For this review, take the finished solid that the model builds, in its own axes (mm). Coordinates: 2 decimals unless noted, no trailing zeros. Loops run counter-clockwise (first coordinate to the right, second up) from the corner with the lowest first, then second, coordinate; pieces in that order, holes last. Notation, with made-up numbers: (67, 24) - (99, 24) arc R24 cw to (99, 58) - close; hole circle Ø5 at (11, 49.25). An arc over 180 degrees is marked (long way). One line per item, written item: value. Start each with the question number.
1. Take a section at B-B, the plane x = 5. Count the separate pieces of the cut face and the enclosed holes in it, and give its area (3 significant figures).
2. Take a section at A-A, the plane y = 31.5. State the section outline as (x, z) points.
3. To check wall thickness, follow line 1 (Y direction, x = -29.5, z = 2.05). State the ranges of the line that lie inside material, in increasing order. Write a range as from..to.
4. Take a section at D-D, the plane x = -28.5. State the section outline as (y, z) points, and give its area (3 significant figures).
5. The part is to be moulded in two halves that separate along Y. For faces 1 (the face through (-5, 49, 1)), 2 (the face through (-15, -58, 1)), say which applies: released by +Y, released by -Y, zero draft, split by the parting line, or undercut.
6. Insertion check: pin 1 (1 mm diameter, centred on x = 25, z = 2.5, fed in from -Y); pin 2 (0.9 mm diameter, centred on y = 58.5, z = 1, fed in from +X). Each pin has a flat end and moves straight along its axis. Give the tip position at first contact, or say it passes through.
```python
from build123d import *

# Parameters (mm, degrees)
SKETCH1_R           = 1.5
BOSS_EXTRUDE1_DEPTH = 3


with BuildPart() as part:
    # Sketch1 → Boss-Extrude1 (new body)
    with BuildSketch(Plane.XY):
        Polygon((-35, 56.5), (-35, -56.5), (-15, -56.5), (-15, -59.5), (15, -59.5), (15, -56.5), (35, -56.5), (35, 56.5), (25, 56.5), (15, 56.5), (15, 59.5), (5, 59.5), (-5, 59.5), (-15, 59.5), (-15, 56.5), (-25, 56.5), align=None)
        with Locations((-25, 51.5)):
            Circle(SKETCH1_R, mode=Mode.SUBTRACT)
        with Locations((-25, 41.5)):
            Circle(SKETCH1_R, mode=Mode.SUBTRACT)
        with Locations((-25, 31.5)):
            Circle(SKETCH1_R, mode=Mode.SUBTRACT)
        with Locations((-25, 21.5)):
            Circle(SKETCH1_R, mode=Mode.SUBTRACT)
        with Locations((-25, 11.5)):
            Circle(SKETCH1_R, mode=Mode.SUBTRACT)
        with Locations((-25, 3.5)):
            Circle(SKETCH1_R, mode=Mode.SUBTRACT)
        with Locations((-25, -3.5)):
            Circle(SKETCH1_R, mode=Mode.SUBTRACT)
        with Locations((-25, -11.5)):
            Circle(SKETCH1_R, mode=Mode.SUBTRACT)
        with Locations((-25, -21.5)):
            Circle(SKETCH1_R, mode=Mode.SUBTRACT)
        with Locations((-25, -31.5)):
            Circle(SKETCH1_R, mode=Mode.SUBTRACT)
        with Locations((-25, -51.5)):
            Circle(SKETCH1_R, mode=Mode.SUBTRACT)
        with Locations((-15, 51.5)):
            Circle(SKETCH1_R, mode=Mode.SUBTRACT)
        with Locations((-15, 41.5)):
            Circle(SKETCH1_R, mode=Mode.SUBTRACT)
        with Locations((-15, 31.5)):
            Circle(SKETCH1_R, mode=Mode.SUBTRACT)
        with Locations((-15, 21.5)):
            Circle(SKETCH1_R, mode=Mode.SUBTRACT)
        with Locations((-15, 11.5)):
            Circle(SKETCH1_R, mode=Mode.SUBTRACT)
        with Locations((-15, 3.5)):
            Circle(SKETCH1_R, mode=Mode.SUBTRACT)
        with Locations((-15, -3.5)):
            Circle(SKETCH1_R, mode=Mode.SUBTRACT)
        with Locations((-15, -11.5)):
            Circle(SKETCH1_R, mode=Mode.SUBTRACT)
        with Locations((-15, -21.5)):
            Circle(SKETCH1_R, mode=Mode.SUBTRACT)
        with Locations((-15, -31.5)):
            Circle(SKETCH1_R, mode=Mode.SUBTRACT)
        with Locations((-15, -51.5)):
            Circle(SKETCH1_R, mode=Mode.SUBTRACT)
        with Locations((-5, 50.5)):
            Circle(SKETCH1_R, mode=Mode.SUBTRACT)
        with Locations((-5, 41.5)):
            Circle(SKETCH1_R, mode=Mode.SUBTRACT)
        with Locations((-5, 31.5)):
            Circle(SKETCH1_R, mode=Mode.SUBTRACT)
        with Locations((-5, 21.5)):
            Circle(SKETCH1_R, mode=Mode.SUBTRACT)
        with Locations((-5, 11.5)):
            Circle(SKETCH1_R, mode=Mode.SUBTRACT)
        with Locations((-5, 3.5)):
            Circle(SKETCH1_R, mode=Mode.SUBTRACT)
        with Locations((-5, -3.5)):
            Circle(SKETCH1_R, mode=Mode.SUBTRACT)
        with Locations((-5, -11.5)):
            Circle(SKETCH1_R, mode=Mode.SUBTRACT)
        with Locations((-5, -21.5)):
            Circle(SKETCH1_R, mode=Mode.SUBTRACT)
        with Locations((-5, -31.5)):
            Circle(SKETCH1_R, mode=Mode.SUBTRACT)
        with Locations((-5, -51.5)):
            Circle(SKETCH1_R, mode=Mode.SUBTRACT)
        with Locations((5, 50.5)):
            Circle(SKETCH1_R, mode=Mode.SUBTRACT)
        with Locations((5, 41.5)):
            Circle(SKETCH1_R, mode=Mode.SUBTRACT)
        with Locations((5, 31.5)):
            Circle(SKETCH1_R, mode=Mode.SUBTRACT)
        with Locations((5, 21.5)):
            Circle(SKETCH1_R, mode=Mode.SUBTRACT)
        with Locations((5, 11.5)):
            Circle(SKETCH1_R, mode=Mode.SUBTRACT)
        with Locations((5, 3.5)):
            Circle(SKETCH1_R, mode=Mode.SUBTRACT)
        with Locations((5, -3.5)):
            Circle(SKETCH1_R, mode=Mode.SUBTRACT)
        with Locations((5, -11.5)):
            Circle(SKETCH1_R, mode=Mode.SUBTRACT)
        with Locations((5, -21.5)):
            Circle(SKETCH1_R, mode=Mode.SUBTRACT)
        with Locations((5, -31.5)):
            Circle(SKETCH1_R, mode=Mode.SUBTRACT)
        with Locations((5, -51.5)):
            Circle(SKETCH1_R, mode=Mode.SUBTRACT)
        with Locations((15, 51.5)):
            Circle(SKETCH1_R, mode=Mode.SUBTRACT)
        with Locations((15, 41.5)):
            Circle(SKETCH1_R, mode=Mode.SUBTRACT)
        with Locations((15, 31.5)):
            Circle(SKETCH1_R, mode=Mode.SUBTRACT)
        with Locations((15, 21.5)):
            Circle(SKETCH1_R, mode=Mode.SUBTRACT)
        with Locations((15, 11.5)):
            Circle(SKETCH1_R, mode=Mode.SUBTRACT)
        with Locations((15, 3.5)):
            Circle(SKETCH1_R, mode=Mode.SUBTRACT)
        with Locations((15, -3.5)):
            Circle(SKETCH1_R, mode=Mode.SUBTRACT)
        with Locations((15, -11.5)):
            Circle(SKETCH1_R, mode=Mode.SUBTRACT)
        with Locations((15, -21.5)):
            Circle(SKETCH1_R, mode=Mode.SUBTRACT)
        with Locations((15, -31.5)):
            Circle(SKETCH1_R, mode=Mode.SUBTRACT)
        with Locations((15, -51.5)):
            Circle(SKETCH1_R, mode=Mode.SUBTRACT)
        with Locations((25, 51.5)):
            Circle(SKETCH1_R, mode=Mode.SUBTRACT)
        with Locations((25, 41.5)):
            Circle(SKETCH1_R, mode=Mode.SUBTRACT)
        with Locations((25, 31.5)):
            Circle(SKETCH1_R, mode=Mode.SUBTRACT)
        with Locations((25, 21.5)):
            Circle(SKETCH1_R, mode=Mode.SUBTRACT)
        with Locations((25, 11.5)):
            Circle(SKETCH1_R, mode=Mode.SUBTRACT)
        with Locations((25, 3.5)):
            Circle(SKETCH1_R, mode=Mode.SUBTRACT)
        with Locations((25, -3.5)):
            Circle(SKETCH1_R, mode=Mode.SUBTRACT)
        with Locations((25, -11.5)):
            Circle(SKETCH1_R, mode=Mode.SUBTRACT)
        with Locations((25, -21.5)):
            Circle(SKETCH1_R, mode=Mode.SUBTRACT)
        with Locations((25, -31.5)):
            Circle(SKETCH1_R, mode=Mode.SUBTRACT)
        with Locations((25, -51.5)):
            Circle(SKETCH1_R, mode=Mode.SUBTRACT)
        with Locations((-25, -41.5)):
            Circle(SKETCH1_R, mode=Mode.SUBTRACT)
        with Locations((-15, -41.5)):
            Circle(SKETCH1_R, mode=Mode.SUBTRACT)
        with Locations((-5, -41.5)):
            Circle(SKETCH1_R, mode=Mode.SUBTRACT)
        with Locations((5, -41.5)):
            Circle(SKETCH1_R, mode=Mode.SUBTRACT)
        with Locations((15, -41.5)):
            Circle(SKETCH1_R, mode=Mode.SUBTRACT)
        with Locations((25, -41.5)):
            Circle(SKETCH1_R, mode=Mode.SUBTRACT)
    extrude(amount=BOSS_EXTRUDE1_DEPTH)


solid = part.part
```
Solutions:
1. separate pieces: 13
1. enclosed holes: 0
1. area: 249 mm2
2. outline: (-35, 0) - (-26.5, 0) - (-26.5, 3) - (-35, 3) - close; (-23.5, 0) - (-16.5, 0) - (-16.5, 3) - (-23.5, 3) - close; (-13.5, 0) - (-6.5, 0) - (-6.5, 3) - (-13.5, 3) - close; (-3.5, 0) - (3.5, 0) - (3.5, 3) - (-3.5, 3) - close; (6.5, 0) - (13.5, 0) - (13.5, 3) - (6.5, 3) - close; (16.5, 0) - (23.5, 0) - (23.5, 3) - (16.5, 3) - close; (26.5, 0) - (35, 0) - (35, 3) - (26.5, 3) - close
3. line 1: -56.5..56.5
4. outline: (-56.5, 0) - (56.5, 0) - (56.5, 3) - (-56.5, 3) - close
4. area: 339 mm2
5. face 1: undercut
5. face 2: zero draft
6. pin 1: y = -56.5
6. pin 2: x = 15
